```python
from build123d import *

# Parameters (mm, degrees)
F1_DEPTH   = 1219.2
F2_W       = 23.9416415725
F2_H       = 38.1
F3_DEPTH   = 17.7778808061
F5_D       = 12.7
F7_D       = 12.7
F8_DEPTH   = 18.3432517809
F1_FACE1_W = 24.0414338853
F1_FACE1_H = 1181.1
F9_DEPTH   = 25.4
F10_W      = 23.5252457925
F10_H      = 38.1
F11_DEPTH  = 25.4
F13_DEPTH  = 25.4


with BuildPart() as f1:
    # F0 (on Top) → F1 (new body)
    with BuildSketch(Plane.XY):
        Polygon((0, 76.2), (0, 0), (-12.4657263412, -20.1891490921), (-7.0626754618, -23.5252457925), (5.8765254397, -1.6680483502), (5.8765254397, 74.5319516498), (17.7768808061, 95.4214725972), (12.2084825006, 98.4735932223), align=None)
    extrude(amount=-F1_DEPTH)

    # F2 (on Right) → F3 (cut, through all)
    with BuildSketch(Plane.YZ):
        with Locations((86.5027724361, -1200.15)):
            Rectangle(F2_W, F2_H)
    extrude(amount=F3_DEPTH, mode=Mode.SUBTRACT)

    # F5 (through all)
    with Locations(Plane.YZ.offset(5.8765254397)):
        with Locations((55.4819516498, -1200.15), (17.3819516498, -1200.15)):
            Hole(F5_D / 2)

    # F7 (through all)
    with Locations(Plane.YZ.offset(5.8765254397)):
        with Locations((55.4819516498, -38.1), (17.3819516498, -38.1)):
            Hole(F7_D / 2)

    # F4 (on face) → F8 (cut, through all)
    with BuildSketch(Plane.YZ.offset(5.8765254397)):
        Polygon((98.4861776233, 0), (74.5319516498, 0), (98.4861776233, -25.4), align=None)
        Polygon((-22.3291479051, 0), (-22.3291479051, -25.4), (-1.6680483502, 0), align=None)
    extrude(amount=-F8_DEPTH, mode=Mode.SUBTRACT)

    # F4 (on face) + F1_face1 (on face) → F9 (cut)
    with BuildSketch(Plane.YZ.offset(5.8765254397)):
        Polygon((98.4861776233, 0), (74.5319516498, 0), (98.4861776233, -25.4), align=None)
        Polygon((-22.3291479051, 0), (-22.3291479051, -25.4), (-1.6680483502, 0), align=None)
    with BuildSketch(Plane(origin=(11.8267031229, 84.9767121235, -590.55), x_dir=(0.4949935775, 0.8688966327, 0), z_dir=(0.8688966327, -0.4949935775, 0))):
        Rectangle(F1_FACE1_W, F1_FACE1_H)
    extrude(amount=F9_DEPTH, dir=(1, 0, 0), mode=Mode.SUBTRACT)

    # F10 (on face) → F11 (cut)
    with BuildSketch(Plane.YZ.offset(5.8765254397)):
        with Locations((-11.7626228962, -1200.15)):
            Rectangle(F10_W, F10_H)
    extrude(amount=-F11_DEPTH, mode=Mode.SUBTRACT)

    # F12 (on face) → F13 (cut)
    with BuildSketch(Plane.YZ.offset(5.8765254397)):
        Polygon((0, -746.356010437), (0, 0), (-23.5252457925, 0), (-23.5252457925, -746.356010437), (-23.5252457925, -819.4740414619), align=None)
    extrude(amount=-F13_DEPTH, mode=Mode.SUBTRACT)


solid = f1.part
```
For this review, take the finished solid that the model builds, in its own axes (mm). A direction names the side the tool comes from. Round coordinates to 2 decimals unless told otherwise and drop trailing zeros. Write each loop counter-clockwise with the first axis right and the second up, starting at its lowest first coordinate (ties: lowest second). Pieces come first, ordered by that corner, then holes.
1) Take a section at B-B on z = -282. Give the boundary of the cut face in (x, y), then the cut area to 3 significant figures.
Answer below:
outline: (0, 0) - (5.88, 0) - (5.88, 74.53) - (17.78, 95.42) - (12.21, 98.47) - (0, 76.2) - close
area: 595 mm2
2) For line 1 along Y through (x, z) = (2.8, -1200.15); line 2 along Z through (x, y) = (5.5, 17); line 3 along X through (y, z) = (50, -690), list the stretches that pass through material, from the lowest coordinate up.
Answer below:
line 1: y = 0 to 11.03, 23.73 to 49.13, 61.83 to 74.53
line 2: z = -1219.2 to -1206.49, -1193.81 to -44.44, -31.76 to 0
line 3: x = 0 to 5.88
3) Machinability: for faces 1 (the face through (9.01, 86.34, -12.52)), 2 (the face through (5.877, 36, -601)), 3 (the face through (0, 39, -601)), which of the approach directions +Z, -Z, +X, -X, +Y, -Y give a long, thin tool a straight path to every point of the face, cutting with its end or side? Answer none if there is none.
Answer below:
face 1: +Z, +X, -X, +Y
face 2: +Z, -Z, +X, -Y
face 3: +Z, -Z, -X, +Y
4) Insertion check: pin 1 Ø23 at (y, z) = (36.5, -404) entering from -X; pin 2 Ø16.5 at (y, z) = (55.48, -38.1) entering from +X; pin 3 Ø8 at (x, y) = (11, 51) entering from +Z; pin 4 Ø12 at (x, z) = (7, -880.5) entering from +Y. Each pin has a flat end and moves straight along its axis. Give the tip position at first contact, or say it passes through.
Answer below:
pin 1: stops at x = 0
pin 2: stops at x = 5.88
pin 3: passes through
pin 4: stops at y = 98.47
5) Take a section at A-A on z = -1084. Give the boundary of the cut face in (x, y), then the cut area to 3 significant figures.
Answer below:
outline: (-12.47, -20.19) - (-7.06, -23.53) - (5.88, -1.67) - (5.88, 74.53) - (17.78, 95.42) - (12.21, 98.47) - (0, 76.2) - (0, 0) - close
area: 750 mm2
